The drawing under review shows one solid part. Ordinate dimensions are in mm from its lowest x, y, z. A direction names the side the tool comes from. Coordinates: 2 decimals unless noted, no trailing zeros. Order: outer loops, then holes, each group sorted by start corner. A loop starts at its lowest first (then second) coordinate and runs counter-clockwise, first axis right, second up.
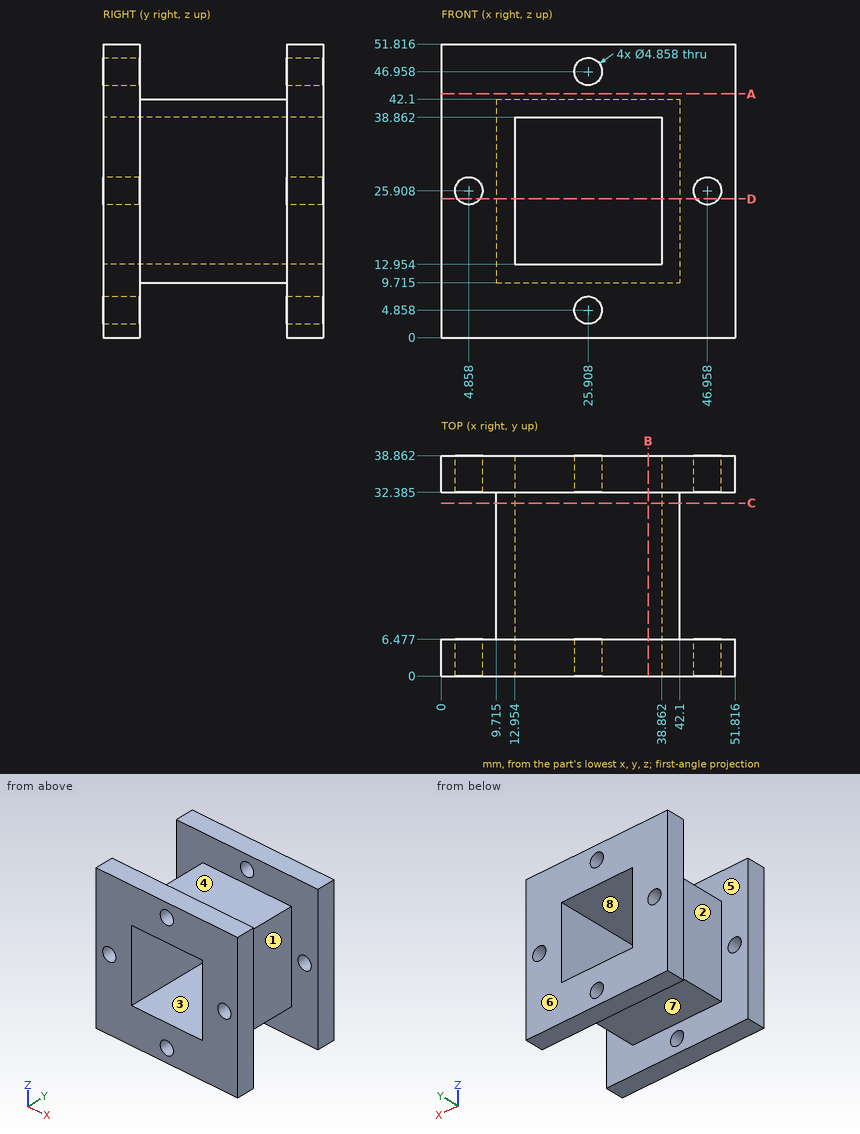
1. To check wall thickness, follow L1, parallel to Y at x = 7, z = 24 (1 decimal); L2, parallel to Z at x = 22, y = 16.5 (1 decimal). State the ranges of each line that lie inside material, in increasing order.
Answer below:
L1: y = 0 to 6.5, 32.4 to 38.9
L2: z = 9.7 to 13, 38.9 to 42.1
2. Take a section at A-A, the plane z = 43. Give the boundary of the cut face in (x, y) (1 decimal), plus the area to 3 significant figures.
Answer below:
outline: (0, 0) - (51.8, 0) - (51.8, 6.5) - (0, 6.5) - close; (0, 32.4) - (51.8, 32.4) - (51.8, 38.9) - (0, 38.9) - close
area: 671 mm2
3. Take a section at C-C, the plane y = 30.5. Give the boundary of the cut face in (x, z) (1 decimal).
Answer below:
outline: (9.7, 9.7) - (42.1, 9.7) - (42.1, 42.1) - (9.7, 42.1) - close; hole (13, 13) - (38.9, 13) - (38.9, 38.9) - (13, 38.9) - close
4. Take a section at D-D, the plane z = 24.5. Give the number of separate pieces and of enclosed holes in the cut face, plus the area to 3 significant figures.
Answer below:
separate pieces: 6
enclosed holes: 0
area: 401 mm2
5. Machinability: for the marked faces 1, 2, 3, 4 and 5, which of the approach directions +Z, -Z, +X, -X, +Y, -Y give a long, thin tool a straight path to every point of the face, cutting with its end or side? Answer none if there is none.
Answer below:
face 1: +Z, -Z, +X
face 2: +Z, -Z, -X
face 3: +Y, -Y
face 4: +Z, +X, -X
face 5: none
6. The part is to be moulded in two halves that separate along Z. For the marked faces 6, 7 and 8, say which applies: +Z half, -Z half, draft (parallel to the pull), parting line (faces both ways), or undercut.
Answer below:
face 6: draft
face 7: -Z half
face 8: undercut
7. Clearance check with flat-ended pins moving along their axes: pin 1 Ø20.5 at (y, z) = (18, 27) entering from +X; pin 2 Ø6 at (x, y) = (38.5, 14.5) entering from -Z (1 decimal); pin 3 Ø2 at (x, z) = (33, 15) entering from +Y; pin 4 Ø13 at (y, z) = (24, 21) entering from -X (1 decimal). State where each tip first meets the part, or that it passes through.
Answer below:
pin 1: stops at x = 42.1
pin 2: stops at z = 9.7
pin 3: passes through
pin 4: stops at x = 9.7
8. Take a section at B-B, the plane x = 36.5. Give the boundary of the cut face in (y, z) (1 decimal).
Answer below:
outline: (0, 0) - (6.5, 0) - (6.5, 9.7) - (32.4, 9.7) - (32.4, 0) - (38.9, 0) - (38.9, 13) - (0, 13) - close; (0, 38.9) - (38.9, 38.9) - (38.9, 51.8) - (32.4, 51.8) - (32.4, 42.1) - (6.5, 42.1) - (6.5, 51.8) - (0, 51.8) - close
